Autodesk Inventor part; units mm, degrees
ref_plane "YZ Plane" through (0, 0, 0) normal (1, 0, 0) x (0, 1, 0)
ref_plane "XZ Plane" through (0, 0, 0) normal (0, 1, 0) x (-1, 0, 0)
ref_plane "XY Plane" through (0, 0, 0) normal (0, 0, 1) x (1, 0, 0)
sketch "Esquisse1" plane through (0, 0, 0) normal (0, 1, 0) x (-1, 0, 0)
  line L0 (7.7669, 22.1799) -> (-26.2331, 22.1799)
  line L1 (-26.2331, 22.1799) -> (-26.2331, -11.8201)
  line L2 (-26.2331, -11.8201) -> (7.7669, -11.8201)
  line L3 (7.7669, -11.8201) -> (7.7669, 22.1799)
  point P0 (0, 0)
  dimension "d0" = 34
  dimension "d1" = 34
extrude "Extrusion1" add sketch "Esquisse1" along normal blind 9
sketch "Esquisse2" plane through (0, 9, 0) normal (0, 1, 0) x (1, 0, 0)
  circle A0 centre (-2.7669, -17.1799) radius 1.5
  circle A1 centre (21.2331, 6.8201) radius 1.5
  line L0 (-7.7669, 11.8201) -> (-7.7669, -22.1799)
  line L1 (-7.7669, -22.1799) -> (26.2331, -22.1799)
  line L2 (26.2331, 11.8201) -> (-7.7669, 11.8201)
  line L3 (26.2331, -22.1799) -> (26.2331, 11.8201)
  point P0 (0, 0)
  dimension "d4" = 3
  dimension "d5" = 3
  dimension "d6" = 5
  dimension "d8" = 5
  dimension "d9" = 5
  dimension "d13" = 5
extrude "Extrusion2" cut sketch "Esquisse2" against normal blind 10 contours A0 | A1
fillet "Congé1" radius 1 12 edges at (9.2331, 9, 22.1799) (26.2331, 9, 5.1799) (9.2331, 9, -11.8201) (-7.7669, 9, 5.1799) (-7.7669, 0, 5.1799) (9.2331, 0, -11.8201) (26.2331, 0, 5.1799) (9.2331, 0, 22.1799) (26.2331, 4.5, 22.1799) (26.2331, 4.5, -11.8201) (-7.7669, 4.5, -11.8201) (-7.7669, 4.5, 22.1799)
properties part number "calle-patin"
Geometry check sheet. Reference: the model listing, model coordinates, mm. Give positions to 0.01 mm unless a question says otherwise; leave off trailing zeros. Write each loop counter-clockwise with the first axis right and the second up, starting at its lowest first coordinate (ties: lowest second). Pieces come first, ordered by that corner, then holes. Notation, with made-up numbers: M -18.5,-36 L 33.5,-36 A34 cw 33.5,-5 Z; hole C 40.25,53 d3. An arc over 180 degrees is marked long. Answer as CSV lines item,"result". Start each with the question number.
Q1. Material ranges on L1, parallel to X at y = 0.5, z = -6.5; L2, parallel to X at y = 2.75, z = -7; L3, parallel to Z at x = -1.5, y = 8.25, recorded low to high.
Q2. Release check for a two-part mould opening along X. For faces 1 (the face through (-3.9, 4.6, 16.2)), 2 (the face through (9.457, 8.715, 21.879)), 3 (the face through (25.95, 4.55, -11.52)) record: pulls with the +X half, pulls with the -X half, needs draft (parallel to the pull), parting line crosses it, or undercut.
Q3. Section check A-A, the plane x = -2.5. Record the cut outline in (y, z).
Q4. Go/stop test with flat-tipped pins: pin 1 (2.5 mm diameter, centred on x = 21.23, z = -6.82, fed in from +Y); pin 2 (3 mm diameter, centred on x = 7, z = 12, fed in from -Y). Record where each tip stops, or that it passes through.
Geometry says:
1,L1,"-7.63 to 19.77, 22.7 to 26.1"
1,L2,"-7.77 to 19.74, 22.72 to 26.23"
1,L3,"-11.79 to 16.38, 17.98 to 22.15"
2,face 1,"undercut"
2,face 2,"needs draft"
2,face 3,"pulls with the +X half"
3,outline,"M 0,-10.82 A1 ccw 1,-11.82 L 8,-11.82 A1 ccw 9,-10.82 L 9,15.7 L 0,15.7 Z; M 0,18.66 L 9,18.66 L 9,21.18 A1 ccw 8,22.18 L 1,22.18 A1 ccw 0,21.18 Z"
4,pin 1,"through"
4,pin 2,"y = 0"
